Autodesk Fusion 360 part; units mm, degrees
sketch "Sketch1" plane through (0, 0, 0) normal (0, 1, 0) x (1, 0, 0)
  line L0 (0, 0) -> (47, 0) construction
  line L1 (47, 0) -> (47, 20.5) construction
  line L2 (47, 20.5) -> (0, 20.5) construction
  line L3 (0, 20.5) -> (0, 0) construction
  line L4 (-0.5, -0.5) -> (47.5, -0.5)
  line L5 (47.5, -0.5) -> (47.5, 21)
  line L6 (47.5, 21) -> (-0.5, 21)
  line L7 (-0.5, 21) -> (-0.5, -0.5)
  dimension "d1" = 47
  dimension "d2" = 20.5
  dimension "d3" = 0.5
extrude "Extrude1" add sketch "Sketch1" along normal blind 25 makes body 1
copy_body "Body->Comp1" bodies 1 removing the originals makes body 2 in component "ServoMount"
shell "Shell1" thickness 2 outward yes removed faces 0 bodies 2 in component "ServoMount"
extrude "Extrude1'" cut 1 faces at (14.8333, 27, -14.5) along direction (0, -1, 0) blind 2 on bodies 2 bodies 2 in component "ServoMount"
ref_plane "WorkPlane1" through (-2.5, 11.5, -10.25) normal (-1, 0, 0) x (0, 0, 1)
sketch "Sketch2" plane through (-2.5, 11.5, -10.25) normal (-1, 0, 0) x (0, 0, -1) in component "ServoMount"
  line L0 (-12.75, -13.5) -> (-8.75, -13.5)
  line L1 (-8.75, -13.5) -> (-8.75, 13.5)
  line L2 (-8.75, 13.5) -> (-12.75, 13.5)
  line L3 (-12.75, 13.5) -> (-12.75, -13.5)
  point P0 (-12.75, -13.5)
  dimension "d10" = 4
extrude "Extrude2" add sketch "Sketch2" along normal blind 20 bodies 2 in component "ServoMount"
ref_plane "WorkPlane2" through (-12.5, 11.5, -1.5) normal (0, 0, -1) x (0, -1, 0) in component "ServoMount"
sketch "Sketch3" plane through (-12.5, 11.5, -1.5) normal (0, 0, -1) x (1, 0, 0) in component "ServoMount"
  circle A0 centre (0, -7) radius 1.5
  line L0 (10, -13.5) -> (-10, -13.5)
  line L1 (-10, -13.5) -> (-10, 13.5)
  circle A1 centre (0, 7) radius 1.5
  line L2 (10, 13.5) -> (-10, 13.5)
  circle A2 centre (0, -7) radius 2.5
  circle A3 centre (0, 7) radius 2.5
  dimension "d14" = 3
  dimension "d15" = 6.5
  dimension "d16" = 10
  dimension "d17" = 3
  dimension "d18" = 10
  dimension "d19" = 6.5
  dimension "d24" = 1
  dimension "d25" = 1
extrude "Extrude3" cut sketch "Sketch3" against normal up to surface (4 mm away) contours A0 bodies 2 in component "ServoMount"
extrude "Extrude4" cut sketch "Sketch3" against normal up to surface (4 mm away) contours A1 bodies 2 in component "ServoMount"
extrude "Extrude5" cut sketch "Sketch3" against normal blind 1 contours A2 bodies 2 in component "ServoMount"
extrude "Extrude6" cut sketch "Sketch3" against normal blind 1 contours A3 bodies 2 in component "ServoMount"
component "ServoMount" placed x (1, 0, 0) y (0, 1, 0) z (0, 0, 1) at (0, 0, 0)
Can you work these out from the model? Positions are in its coordinate system, mm. A direction names the side the tool comes from. Round coordinates to 2 decimals unless told otherwise and drop trailing zeros. Loops run counter-clockwise (first coordinate to the right, second up) from the corner with the lowest first, then second, coordinate; pieces in that order, holes last.
Item 1: Suppose I cut it at D-D, the plane z = -12. Write out the boundary of the cut face in (x, y), then the cut area to 3 significant figures.
Item 2: Suppose I cut it at C-C, the plane y = 13.75. Write out the boundary of the cut face in (x, z).
Item 3: If we mould it in two halves opening along Y, with no side actions, what happens to faces 1 (the flat face through (-22.5, 11, 1)), 2 (the cylindrical face through (-15, 18.4, -1)), 3 (the flat face through (22, 25, -10)), 4 (the flat face through (22, -2, -10))? For each: +Y half, -Y half, draft (parallel to the pull), parting line (faces both ways), or undercut.
Item 4: Please list where these lines run through material, in increasing order: L1, parallel to Y at x = -12.5, z = -0.75; L2, parallel to Y at x = -12.5, z = 1.3; L3, parallel to X at y = 4.5, z = 0.5.
Item 5: Will these pins go through, and if not, where does the flat tip stop? pin 1 Ø4 at (y, z) = (14, -12.5) entering from -X; pin 2 Ø1 at (x, y) = (-5, 14) entering from -Z; pin 3 Ø6.5 at (x, y) = (-12.5, 18.5) entering from +Z.
Item 6: Which directions (+Z, -Z, +X, -X, +Y, -Y) give clear straight access to the entire face, cutting with the end or side of a thin tool? Please do faces 5 (the flat face through (-11, 20, -0.5)), 6 (the flat face through (24, 11, -23)), 7 (the flat face through (-12, 12, -1.5)).
Item 7: Suppose I cut it at B-B, the plane x = -12.5. Write out the boundary of the cut face in (y, z), then the cut area to 3 significant figures.
Item 8: Suppose I cut it at A-A, the plane y = 4.5. Write out the boundary of the cut face in (x, z), then the cut area to 3 significant figures.
Reported:
1. outline: (-2.5, -2) - (49.5, -2) - (49.5, 25) - (-2.5, 25) - close
1. area: 1,400 mm2
2. outline: (-22.5, -1.5) - (-2.5, -1.5) - (-2.5, -23) - (49.5, -23) - (49.5, 2.5) - (-22.5, 2.5) - close
3. face 1: draft
3. face 2: undercut
3. face 3: +Y half
3. face 4: -Y half
4. L1: y = -2 to 2, 7 to 16, 21 to 25
4. L2: y = -2 to 3, 6 to 17, 20 to 25
4. L3: x = -22.5 to -14, -11 to 49.5
5. pin 1: stops at x = -2.5
5. pin 2: stops at z = -1.5
5. pin 3: stops at z = 2.5
6. face 5: -Z
6. face 6: -Z, +X, -X, +Y, -Y
6. face 7: -Z, -X, +Y, -Y
7. outline: (-2, -1.5) - (2, -1.5) - (2, -0.5) - (3, -0.5) - (3, 2.5) - (-2, 2.5) - close; (6, -0.5) - (7, -0.5) - (7, -1.5) - (16, -1.5) - (16, -0.5) - (17, -0.5) - (17, 2.5) - (6, 2.5) - close; (20, -0.5) - (21, -0.5) - (21, -1.5) - (25, -1.5) - (25, 2.5) - (20, 2.5) - close
7. area: 80.0 mm2
8. outline: (-22.5, -1.5) - (-15, -1.5) - (-15, -0.5) - (-14, -0.5) - (-14, 2.5) - (-22.5, 2.5) - close; (-11, -0.5) - (-10, -0.5) - (-10, -1.5) - (-2.5, -1.5) - (-2.5, -23) - (49.5, -23) - (49.5, 2.5) - (-11, 2.5) - close
8. area: 1,390 mm2
